Drawing for the job (mm, zero at the part's lowest x, y, z). A direction names the side the tool comes from. Coordinates: 2 decimals unless noted, no trailing zeros. Write each loop counter-clockwise with the first axis right and the second up, starting at its lowest first coordinate (ties: lowest second). Pieces come first, ordered by that corner, then holes. Notation, with made-up numbers: (83, 63.25) -> (94, 63.25) arc R30 ccw to (94, 102.25) -> close; hole circle Ø6 at (36.25, -25). An arc over 180 degrees is marked (long way). Answer as CSV lines item,"result".
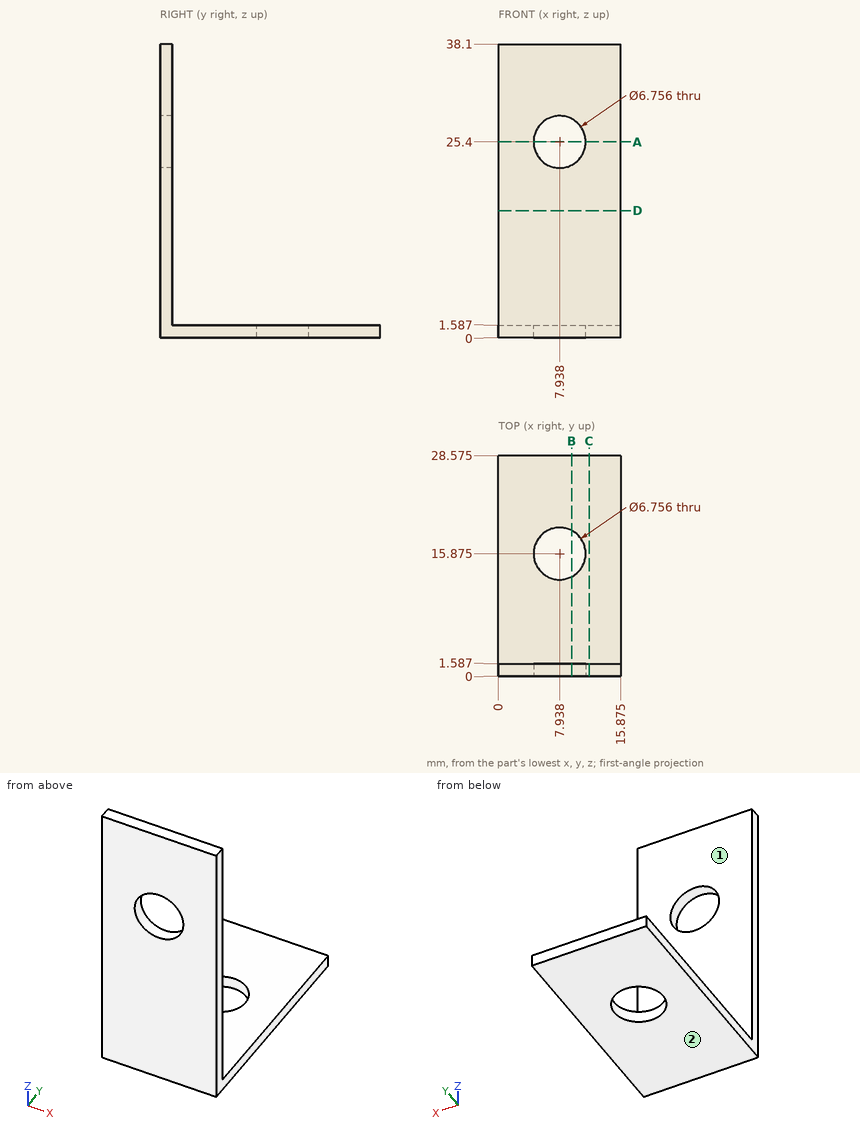
Item 1: Wall check: line 1 (Z direction, x = 9.5, y = 26.25); line 2 (X direction, y = 0.65, z = 25.4) (1 decimal). Give the ranges that are in metal, low to high. Write a range as from..to.
Answer below:
line 1,"z = 0..1.59"
line 2,"x = 0..4.6, 11.3..15.9"
Item 2: Saw through at B-B on x = 9.5. Give the cut face in (y, z) (1 decimal).
Answer below:
outline,"(0, 0) -> (12.9, 0) -> (12.9, 1.6) -> (1.6, 1.6) -> (1.6, 22.4) -> (0, 22.4) -> close; (0, 28.4) -> (1.6, 28.4) -> (1.6, 38.1) -> (0, 38.1) -> close; (18.9, 0) -> (28.6, 0) -> (28.6, 1.6) -> (18.9, 1.6) -> close"
Item 3: Saw through at D-D on z = 16.5. Give the cut face in (x, y) (1 decimal).
Answer below:
outline,"(0, 0) -> (15.9, 0) -> (15.9, 1.6) -> (0, 1.6) -> close"
Item 4: 3-axis set-ups, long thin cutter, end or side, ignore diameter. For the marked faces 1 and 2: which of +Z, -Z, +X, -X, +Y, -Y reach the whole face in a straight line?
Answer below:
face 1,"+Z, +X, -X, +Y"
face 2,"-Z, +X, -X, +Y, -Y"
Item 5: Saw through at A-A on z = 25.4. Give the cut face in (x, y) (1 decimal), and give its area (3 significant figures).
Answer below:
outline,"(0, 0) -> (4.6, 0) -> (4.6, 1.6) -> (0, 1.6) -> close; (11.3, 0) -> (15.9, 0) -> (15.9, 1.6) -> (11.3, 1.6) -> close"
area,"14.5 mm2"
Item 6: Flat gauge pins, fed straight in: pin 1 (8 mm diameter, centred on x = 8, z = 24.5, fed in from +Y); pin 2 (5 mm diameter, centred on x = 4, y = 19, fed in from +Z). Where does each tip first touch, or does it go through?
Answer below:
pin 1,"stops at y = 1.59"
pin 2,"stops at z = 1.59"
Item 7: Saw through at C-C on x = 11.75. Give the cut face in (y, z) (1 decimal), and give its area (3 significant figures).
Answer below:
outline,"(0, 0) -> (28.6, 0) -> (28.6, 1.6) -> (1.6, 1.6) -> (1.6, 38.1) -> (0, 38.1) -> close"
area,"103 mm2"
